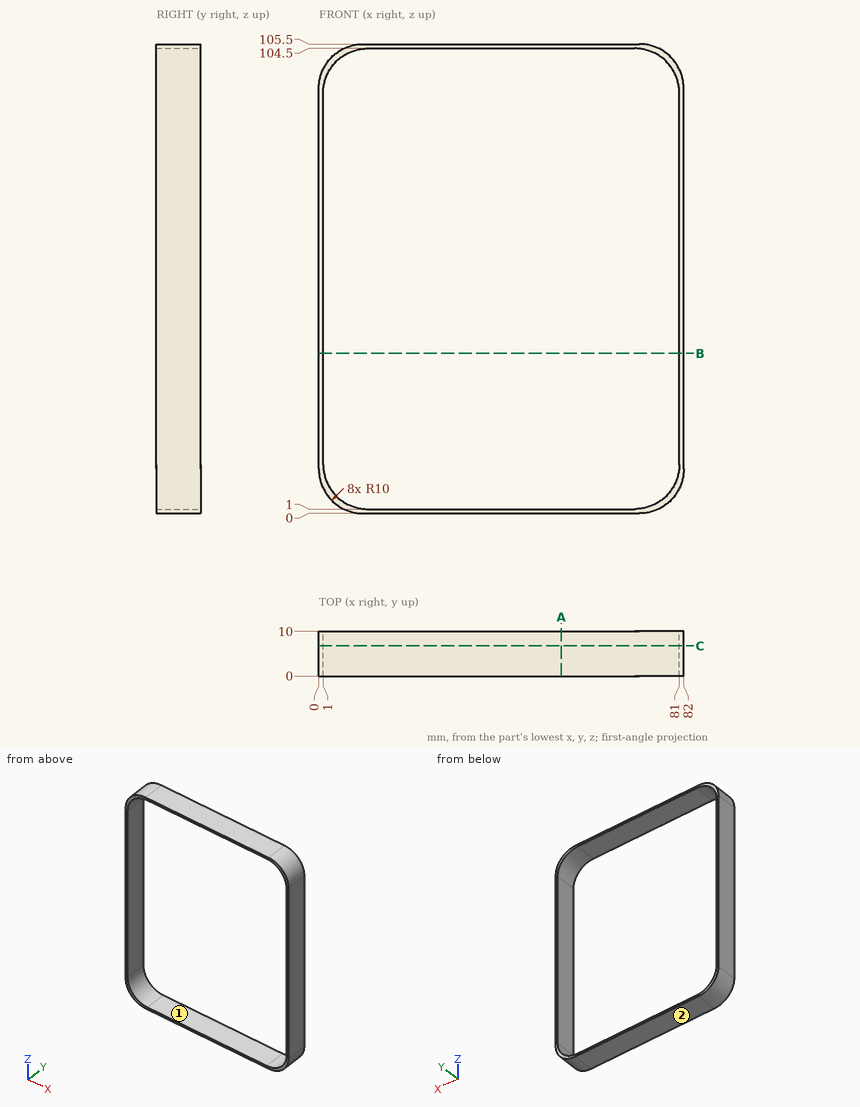
Can you work these out from the drawing? Everything is in mm from the part's minimum corner. A direction names the side the tool comes from. Give positions to 0.01 mm unless a question says otherwise; leave off trailing zeros. Order: outer loops, then holes, each group sorted by start corner. A loop starts at its lowest first (then second) coordinate and runs counter-clockwise, first axis right, second up. Notation, with made-up numbers: M 7,-13.5 L 27,-13.5 A20 cw 27,11.5 Z; hole C 88,47 d9. An arc over 180 degrees is marked long. Use a Markdown table: item, result. Add a question column.
Item 1: Suppose I cut it at C-C (y = 6.75). List the corners of the cut face in (x, z) for me, then the cut area to 3 significant figures.
Item 2: Suppose I cut it at A-A (x = 54.5). List the corners of the cut face in (y, z) for me, then the cut area to 3 significant figures.
Item 3: Will this pin go through, and if not, where does the flat tip stop? pin 1 (4 mm diameter, centred on y = 3, z = 46, fed in from -X).
Item 4: For the marked faces 1 and 2, which set-ups out of +Z, -Z, +X, -X, +Y, -Y let a thin tool reach every point of the face, with its end or its side?
Item 5: Suppose I cut it at B-B (z = 36). List the corners of the cut face in (x, y) for me, then the cut area to 3 significant figures.
Item 6: If I drill on L1, parallel to Z at x = 33.5, y = 8.5; L2, parallel to X at y = 4.5, z = 54.5; L3, parallel to Z at x = 72.5, y = 0.75, over which ranges is the centre line in solid material (lowest first)? Write a range as [from, to].
Answer sheet:
| question | item | result |
|---|---|---|
| 1 | outline | M 0,10 A10 ccw 10,0 L 72,0 A10 ccw 82,10 L 82,95.5 A10 ccw 72,105.5 L 10,105.5 A10 ccw 0,95.5 Z; hole M 1,11 A10 ccw 11,1 L 71,1 A10 ccw 81,11 L 81,94.5 A10 ccw 71,104.5 L 11,104.5 A10 ccw 1,94.5 Z |
| 1 | area | 371 mm² |
| 2 | outline | M 0,0 L 10,0 L 10,1 L 0,1 Z; M 0,104.5 L 10,104.5 L 10,105.5 L 0,105.5 Z |
| 2 | area | 20.0 mm² |
| 3 | pin 1 | stops at x = 0 |
| 4 | face 1 | +Y, -Y |
| 4 | face 2 | -Z, +X, -X, +Y, -Y |
| 5 | outline | M 0,0 L 1,0 L 1,10 L 0,10 Z; M 81,0 L 82,0 L 82,10 L 81,10 Z |
| 5 | area | 20.0 mm² |
| 6 | L1 | z = [0, 1], [104.5, 105.5] |
| 6 | L2 | x = [0, 1], [81, 82] |
| 6 | L3 | z = [0.01, 1.11], [104.39, 105.49] |
